Work out the finished part from the listing and answer in its coordinate system (mm). Face numbers are marked on the shaded views. A direction names the side the tool comes from. Round coordinates to 2 decimals unless told otherwise and drop trailing zeros. Write each loop counter-clockwise with the first axis right and the second up, starting at its lowest first coordinate (ties: lowest second). Pieces come first, ordered by that corner, then holes. Notation, with made-up numbers: M -3.5,-15.75 L 13.5,-15.75 A27 cw 13.5,11.25 Z; hole C 46,62.25 d10. An arc over 180 degrees is marked long. Answer in a Markdown table with one row per item.
```python
from build123d import *


with BuildPart() as f1:
    # F0 (on Top) → F1 (revolve)
    with BuildSketch(Plane.XY):
        with BuildLine():
            Line((0, 10.332034), (0, 0))
            Line((0, 0), (15, 0))
            Line((15, 0), (15, 1.8))
            ThreePointArc((15, 1.8), (14.575736, 1.975736), (14.4, 2.4))
            ThreePointArc((14.4, 2.4), (14.575736, 2.824264), (15, 3))
            Line((15, 3), (51.737146, 3))
            Line((51.737146, 3), (67.159845, 6.093667))
            Line((67.159845, 6.093667), (75.813033, 6.093667))
            Line((75.813033, 6.093667), (75.813033, 16.841185))
            Line((75.813033, 16.841185), (49.37445, 16.841185))
            Line((49.37445, 16.841185), (49.37445, 12.015897))
            Line((49.37445, 12.015897), (3.78983, 12.015897))
            Line((3.78983, 12.015897), (0, 10.332034))
        make_face()
    revolve(axis=Axis((26.506836, -21.1, 0), (1, 0, 0)))


solid = f1.part
```
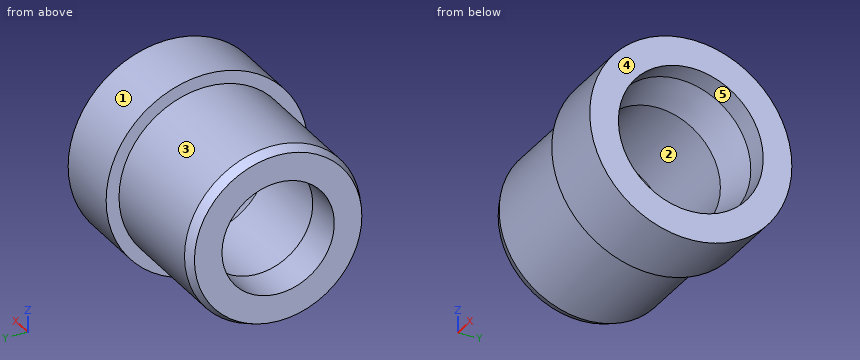
1. The part is cut by section A-A (x = 17). Determine the outline of the cut face in (y, z).
Calculated:
| item | result |
|---|---|
| outline | C -21.1,0 d66.23; hole C -21.1,0 d48.2 |
2. Determine the mould class of the marked faces 3, 4 and 5 for opening direction Y: released by +Y, released by -Y, zero draft, split by the parting line, or undercut.
Calculated:
| item | result |
|---|---|
| face 3 | split by the parting line |
| face 4 | zero draft |
| face 5 | undercut |
3. Consider line 1 along Z through (x, y) = (6, -21); line 2 along Z through (x, y) = (71.5, -21.1); line 3 along Y through (x, z) = (33.5, -12). Determine where each line is inside the solid, lowest interval first. Write a range as from..to.
Calculated:
| item | result |
|---|---|
| line 1 | z = -33.12..-21.1, 21.1..33.12 |
| line 2 | z = -37.94..-27.19, 27.19..37.94 |
| line 3 | y = -51.97..-42, -0.2..9.77 |
4. Given pin 1 (12 mm diameter, centred on y = -33, z = -3, fed in from -X); pin 2 (6 mm diameter, centred on x = 53.5, y = 5, fed in from +Z); pin 3 (12 mm diameter, centred on y = -51, z = -25.5, fed in from -X); pin 4 (3 mm diameter, centred on x = 22.5, z = 26.5, fed in from -Y), each flat-ended and moving along its own axis, determine where each tip first touches the part or whether it passes through.
Calculated:
| item | result |
|---|---|
| pin 1 | passes through |
| pin 2 | stops at z = 30.1 |
| pin 3 | stops at x = 49.37 |
| pin 4 | stops at y = -42.82 |
5. A tool of negligible diameter and unlimited length cuts with its end or side. For the marked faces 1 and 2, from which of +Z, -Z, +X, -X, +Y, -Y can it reach the whole face along a straight path? Write none if from no direction.
Calculated:
| item | result |
|---|---|
| face 1 | +X, -X |
| face 2 | +X |
